from build123d import *

# Parameters (mm, degrees)
F0_W      = 100
F0_H      = 100
F1_DEPTH  = 10
F2_W      = 20
F2_H      = 10
F3_DEPTH  = 10
F4_W      = 20
F4_H      = 10
F5_DEPTH  = 10
F6_W      = 20
F6_H      = 10
F7_DEPTH  = 10
F8_W      = 10
F8_H      = 10
F9_DEPTH  = 10
F10_W     = 10
F10_H     = 10
F11_DEPTH = 10
F12_W     = 10
F12_H     = 10
F13_DEPTH = 10
F14_W     = 10
F14_H     = 10
F15_DEPTH = 10
F16_W     = 10
F16_H     = 10
F17_DEPTH = 10
F18_W     = 10
F18_H     = 10
F19_DEPTH = 10


with BuildPart() as f1:
    # F0 (on Right) → F1 (new body)
    with BuildSketch(Plane.YZ):
        with Locations((11.134875, 6.03618)):
            Rectangle(F0_W, F0_H)
    extrude(amount=F1_DEPTH)

    # F2 (on face) → F3 (cut)
    with BuildSketch(Plane.YZ.offset(10)):
        with Locations((-18.865125, -38.96382)):
            Rectangle(F2_W, F2_H)
    extrude(amount=-F3_DEPTH, mode=Mode.SUBTRACT)

    # F4 (on face) → F5 (cut)
    with BuildSketch(Plane.YZ.offset(10)):
        with Locations((11.134875, -38.96382)):
            Rectangle(F4_W, F4_H)
    extrude(amount=-F5_DEPTH, mode=Mode.SUBTRACT)

    # F6 (on face) → F7 (cut)
    with BuildSketch(Plane.YZ.offset(10)):
        with Locations((41.134875, -38.96382)):
            Rectangle(F6_W, F6_H)
    extrude(amount=-F7_DEPTH, mode=Mode.SUBTRACT)

    # F8 (on face) → F9 (cut)
    with BuildSketch(Plane.YZ.offset(10)):
        with Locations((-33.865125, -18.96382)):
            Rectangle(F8_W, F8_H)
    extrude(amount=-F9_DEPTH, mode=Mode.SUBTRACT)

    # F10 (on face) → F11 (cut)
    with BuildSketch(Plane.YZ.offset(10)):
        with Locations((-33.865125, 11.03618)):
            Rectangle(F10_W, F10_H)
    extrude(amount=-F11_DEPTH, mode=Mode.SUBTRACT)

    # F12 (on face) → F13 (cut)
    with BuildSketch(Plane.YZ.offset(10)):
        with Locations((-33.865125, 41.03618)):
            Rectangle(F12_W, F12_H)
    extrude(amount=-F13_DEPTH, mode=Mode.SUBTRACT)

    # F14 (on face) → F15 (cut)
    with BuildSketch(Plane.YZ.offset(10)):
        with Locations((56.134875, -18.96382)):
            Rectangle(F14_W, F14_H)
    extrude(amount=-F15_DEPTH, mode=Mode.SUBTRACT)

    # F16 (on face) → F17 (cut)
    with BuildSketch(Plane.YZ.offset(10)):
        with Locations((56.134875, 11.03618)):
            Rectangle(F16_W, F16_H)
    extrude(amount=-F17_DEPTH, mode=Mode.SUBTRACT)

    # F18 (on face) → F19 (cut)
    with BuildSketch(Plane.YZ.offset(10)):
        with Locations((56.134875, 41.03618)):
            Rectangle(F18_W, F18_H)
    extrude(amount=-F19_DEPTH, mode=Mode.SUBTRACT)


solid = f1.part
For this review, take the finished solid that the model builds, in its own axes (mm). A direction names the side the tool comes from. Round coordinates to 2 decimals unless told otherwise and drop trailing zeros. Loops run counter-clockwise (first coordinate to the right, second up) from the corner with the lowest first, then second, coordinate; pieces in that order, holes last. Notation, with made-up numbers: (-3, 76) - (9, 76) arc R25 ccw to (9, 90) - close; hole circle Ø8 at (-13.5, 80.5). An arc over 180 degrees is marked (long way). Answer as CSV lines item,"result".
(1) Wall thickness on line 1 (Y direction, x = 4.5, z = -39); line 2 (Z direction, x = 6, y = 57); line 3 (Z direction, x = 7, y = 39): over which ranges is each line inside the solid? List them lowest first.
Checked values:
line 1,"y = -38.87 to -28.87, -8.87 to 1.13, 21.13 to 31.13, 51.13 to 61.13"
line 2,"z = -43.96 to -23.96, -13.96 to 6.04, 16.04 to 36.04, 46.04 to 56.04"
line 3,"z = -33.96 to 56.04"
(2) Consider section A-A on y = 55. Give the boundary of the cut face in (x, z), then the cut area to 3 significant figures.
Checked values:
outline,"(0, -43.96) - (10, -43.96) - (10, -23.96) - (0, -23.96) - close; (0, -13.96) - (10, -13.96) - (10, 6.04) - (0, 6.04) - close; (0, 16.04) - (10, 16.04) - (10, 36.04) - (0, 36.04) - close; (0, 46.04) - (10, 46.04) - (10, 56.04) - (0, 56.04) - close"
area,"700 mm2"
(3) Tool access review of faces 1 (the face through (5, 56, -23.964)), 2 (the face through (10, 10, 7)), 3 (the face through (5, -8.865, -39)), 4 (the face through (5, -28.865, 41)): name each direction out of +Z, -Z, +X, -X, +Y, -Y from which nothing blocks a thin tool from reaching the whole face with its end or side.
Checked values:
face 1,"+X, -X, +Y"
face 2,"+Z, -Z, +X, +Y, -Y"
face 3,"-Z, +X, -X"
face 4,"+X, -X, -Y"
(4) Insertion check: P1, Ø2, axis at x = 2.5, z = -18, coming from the +Y side; P2, Ø1, axis at x = 7.5, z = 45, coming from the -Y side. Each pin has a flat end and moves straight along its axis. Give the tip position at first contact, or say it passes through.
Checked values:
P1,"stops at y = 51.13"
P2,"stops at y = -28.87"
(5) Mouldability with a two-part tool opening along Y and no side actions: class faces 5 (the face through (5, 56, -43.964)), 6 (the face through (5, 1.135, -39)), 7 (the face through (5, 61.135, 26)) as +Y half, -Y half, draft (parallel to the pull), parting line (faces both ways), or undercut.
Checked values:
face 5,"draft"
face 6,"undercut"
face 7,"+Y half"
(6) Consider section C-C on z = 38. Give the boundary of the cut face in (x, y).
Checked values:
outline,"(0, -28.87) - (10, -28.87) - (10, 51.13) - (0, 51.13) - close"
(7) Consider section B-B on y = 6. Give the boundary of the cut face in (x, z).
Checked values:
outline,"(0, -33.96) - (10, -33.96) - (10, 56.04) - (0, 56.04) - close"
